from build123d import *

# Parameters (mm, degrees)
F0_R     = 6.35
F1_DEPTH = 7.62
F2_R     = 5.55625
F3_DEPTH = 1.5875
F4_W     = 5.565012
F4_H     = 2.274479
F4_W_2   = 5.057012
F4_H_2   = 1.766479
F5_DEPTH = 2.54


with BuildPart() as f1:
    # F0 (on Front) → F1 (new body)
    with BuildSketch(Plane.XZ):
        Circle(F0_R)
    extrude(amount=F1_DEPTH)

    # F2 (on face) → F3 (cut)
    with BuildSketch(Plane(origin=(0, 0, 0), x_dir=(-1, 0, 0), z_dir=(0, 1, 0))):
        Circle(F2_R)
    extrude(amount=-F3_DEPTH, mode=Mode.SUBTRACT)

    # F4 (on face) → F5 (join)
    with BuildSketch(Plane.XZ.offset(7.62)):
        with Locations((0, 2.855948)):
            Rectangle(F4_W, F4_H)
        with Locations((0, 2.855948)):
            Rectangle(F4_W_2, F4_H_2, mode=Mode.SUBTRACT)
    extrude(amount=F5_DEPTH)


solid = f1.part
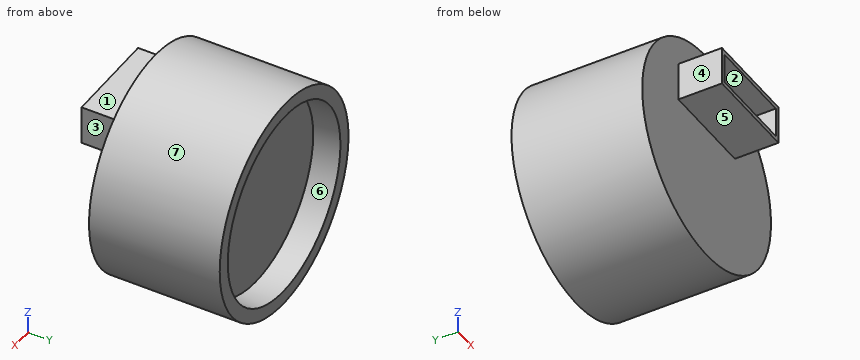
Can you work these out from the model? Positions are in its coordinate system, mm. Face numbers are marked on the shaded views. A direction names the side the tool comes from. Give positions to 0.01 mm unless a question says otherwise; leave off trailing zeros. Write each loop counter-clockwise with the first axis right and the second up, starting at its lowest first coordinate (ties: lowest second). Pieces come first, ordered by that corner, then holes. Notation, with made-up numbers: M 81,21 L 85,21 A3 cw 85,26 Z; hole C 2.25,53 d6. An arc over 180 degrees is marked long. Answer in a Markdown table with one row per item. Add a question column.
Item 1: Please list where these lines run through material, in increasing order: L1, parallel to Z at x = 0, y = -0.5; L2, parallel to X at y = -8.25, z = 3.5; L3, parallel to Y at x = -0.5, z = 3.5.
Item 2: Imagine slicing it at C-C, the plane x = 0. Write out the boundary of the cut face in (y, z).
Item 3: For pin 1 Ø2 at (x, z) = (-2, 3.5) entering from +Y; pin 2 Ø0.8 at (x, y) = (-1, -9) entering from -Z; pin 3 Ø2.5 at (y, z) = (-9.5, 3) entering from +X, each with a flat end and sliding along its axis, tell me the tip position at first contact or that it passes through.
Item 4: On a 3-axis mill with a long thin cutter (end or side, diameter ignored), from which of +Z, -Z, +X, -X, +Y, -Y can I reach the whole of each face in a straight line? I mean the marked faces 4, 5, 6 and 7. Say none if no direction works.
Item 5: We'd pull the mould along X, two halves only. Please class the marked faces 1, 2 and 3: released by +X, released by -X, zero draft, split by the parting line, or undercut.
Item 6: Imagine slicing it at D-D, the plane y = -4. Write out the boundary of the cut face in (x, z).
Item 7: Imagine slicing it at A-A, the plane z = 0. Write out the boundary of the cut face in (x, y), plus the area to 3 significant figures.
Item 8: Imagine slicing it at B-B, the plane y = -8. Write out the boundary of the cut face in (x, z).
Evaluation:
| question | item | result |
|---|---|---|
| 1 | L1 | z = -6.35 to -5.56, 5.56 to 6.35 |
| 1 | L2 | x = -2.78 to -2.53, 2.53 to 2.78 |
| 1 | L3 | y = -7.62 to -1.59 |
| 2 | outline | M -10.16,1.72 L -7.62,1.72 L -7.62,-6.35 L 0,-6.35 L 0,-5.56 L -1.59,-5.56 L -1.59,5.56 L 0,5.56 L 0,6.35 L -7.62,6.35 L -7.62,3.99 L -10.16,3.99 L -10.16,3.74 L -7.62,3.74 L -7.62,1.97 L -10.16,1.97 Z |
| 3 | pin 1 | stops at y = -1.59 |
| 3 | pin 2 | stops at z = 1.72 |
| 3 | pin 3 | stops at x = 2.78 |
| 4 | face 4 | +Z, -Z, -X, -Y |
| 4 | face 5 | -Z, +X, -X, -Y |
| 4 | face 6 | +Y |
| 4 | face 7 | +Y, -Y |
| 5 | face 1 | zero draft |
| 5 | face 2 | undercut |
| 5 | face 3 | released by +X |
| 6 | outline | C 0,0 d12.7 |
| 7 | outline | M -6.35,-7.62 L 6.35,-7.62 L 6.35,0 L 5.56,0 L 5.56,-1.59 L -5.56,-1.59 L -5.56,0 L -6.35,0 Z |
| 7 | area | 79.1 mm² |
| 8 | outline | M -2.78,1.72 L 2.78,1.72 L 2.78,3.99 L -2.78,3.99 Z; hole M -2.53,1.97 L 2.53,1.97 L 2.53,3.74 L -2.53,3.74 Z |
